Verification items for this drawing (mm, ordinates from the low corner). A direction names the side the tool comes from. Give positions to 0.01 mm unless a question says otherwise; leave off trailing zeros. Loops run counter-clockwise (first coordinate to the right, second up) from the corner with the lowest first, then second, coordinate; pieces in that order, holes last. Notation, with made-up numbers: M 28.25,21 L 65.25,21 A19 cw 65.25,28 Z; hole C -20.75,54 d2. An arc over 180 degrees is marked long. Use a Markdown table: item, result.
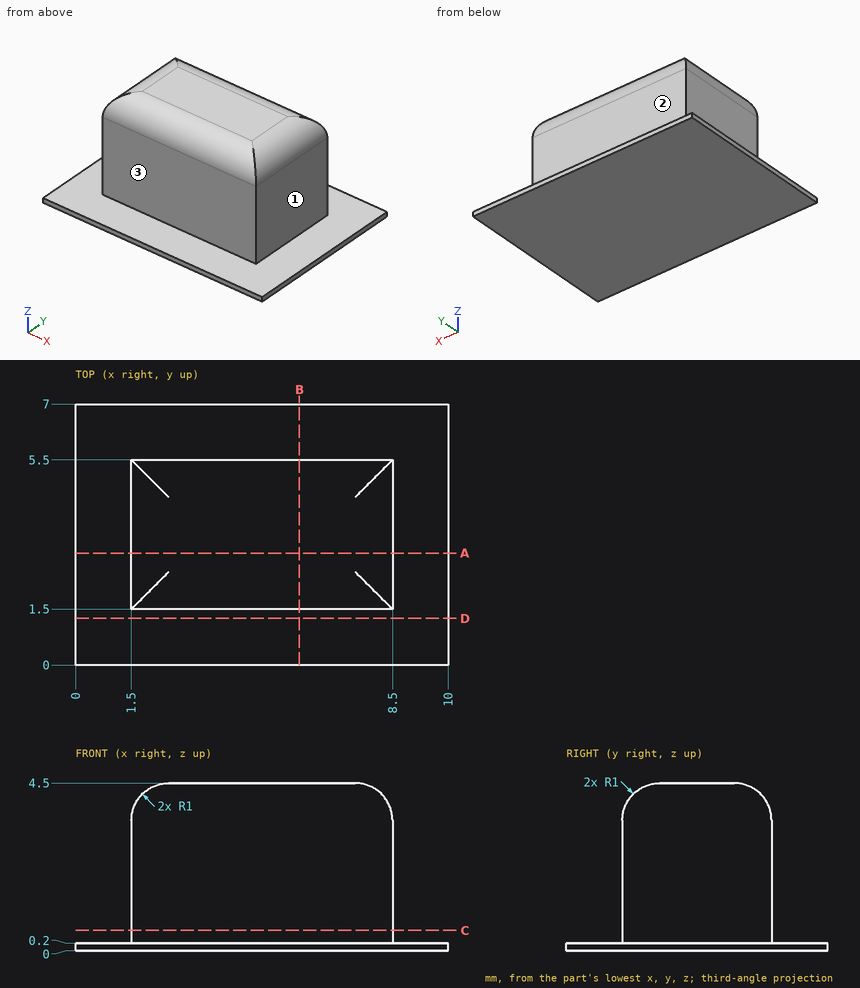
(1) Set-up check for the marked faces 1, 2 and 3: record each of +Z, -Z, +X, -X, +Y, -Y from which the full face is reachable in a straight line by a thin tool's end or side.
Results below:
| item | result |
|---|---|
| face 1 | +Z, +X, +Y, -Y |
| face 2 | +Z, +X, -X, +Y |
| face 3 | +Z, +X, -X, -Y |
(2) Cross-section at A-A on y = 3. Record the cut outline in (x, z), then the cut area to 3 significant figures.
Results below:
| item | result |
|---|---|
| outline | M 0,0 L 10,0 L 10,0.2 L 8.5,0.2 L 8.5,3.5 A1 ccw 7.5,4.5 L 2.5,4.5 A1 ccw 1.5,3.5 L 1.5,0.2 L 0,0.2 Z |
| area | 31.7 mm^2 |
(3) Cross-section at D-D on y = 1.25. Record the cut outline in (x, z).
Results below:
| item | result |
|---|---|
| outline | M 0,0 L 10,0 L 10,0.2 L 0,0.2 Z |
(4) Cross-section at C-C on z = 0.55. Record the cut outline in (x, y), then the cut area to 3 significant figures.
Results below:
| item | result |
|---|---|
| outline | M 1.5,1.5 L 8.5,1.5 L 8.5,5.5 L 1.5,5.5 Z |
| area | 28.0 mm^2 |
(5) Gauge pin test, flat ends, axial feed: P1, Ø1.5, axis at x = 1, z = 1, coming from the -Y side; P2, Ø2.5, axis at y = 2.5, z = 1.5, coming from the -X side; P3, Ø2, axis at x = 6.5, z = 1.5, coming from the +Y side. Record the tip position at first contact, or that the pin passes through.
Results below:
| item | result |
|---|---|
| P1 | y = 1.5 |
| P2 | x = 1.5 |
| P3 | y = 5.5 |
(6) Cross-section at B-B on x = 6. Record the cut outline in (y, z).
Results below:
| item | result |
|---|---|
| outline | M 0,0 L 7,0 L 7,0.2 L 5.5,0.2 L 5.5,3.5 A1 ccw 4.5,4.5 L 2.5,4.5 A1 ccw 1.5,3.5 L 1.5,0.2 L 0,0.2 Z |
(7) Material ranges on line 1 (Z direction, x = 1, y = 5.25); line 2 (X direction, y = 3.75, z = 2.2); line 3 (Y direction, x = 2.5, z = 0.7), recorded low to high.
Results below:
| item | result |
|---|---|
| line 1 | 0 to 0.2 |
| line 2 | 1.5 to 8.5 |
| line 3 | 1.5 to 5.5 |
